```python
from build123d import *
from build123d.topology import SkipClean

# Parameters (mm, degrees)
SKETCH1_R    = 19.05
SKETCH1_R_2  = 12.7
TOP_DEPTH    = 12.7
MIDDLE_START = 6.35
SKETCH4_R    = 28.575
SKETCH4_R_2  = 12.7
MIDDLE_DEPTH = 6.35
BOTTOM_START = 12.7
SKETCH5_R    = 15.875
SKETCH5_R_2  = 12.7
BOTTOM_DEPTH = 12.7


with BuildPart() as part:
    # Sketch1 → Top (new body)
    with BuildSketch(Plane(origin=(0, 0, 0), x_dir=(1, 0, 0), z_dir=(0, 1, 0))):
        with Locations(Location((0, 0, 0), (0, 0, 270))):
            Circle(SKETCH1_R)
        with Locations(Location((0, 0, 0), (0, 0, 270))):
            Circle(SKETCH1_R_2, mode=Mode.SUBTRACT)
    extrude(amount=TOP_DEPTH)

    # Sketch4 → Middle (add)
    with SkipClean():  # the faces are left unmerged after this step: merging them gives an invalid solid
        with BuildSketch(Plane.XZ.offset(MIDDLE_START)):
            with Locations(Location((0, 0, 0), (0, 0, 270))):
                Circle(SKETCH4_R)
            with Locations(Location((0, 0, 0), (0, 0, 270))):
                Circle(SKETCH4_R_2, mode=Mode.SUBTRACT)
        extrude(amount=-MIDDLE_DEPTH)

    # Sketch5 → Bottom (add)
    with SkipClean():  # the faces are left unmerged after this step: merging them gives an invalid solid
        with BuildSketch(Plane.XZ.offset(6.35).offset(BOTTOM_START)):
            with Locations(Location((0, 0, 0), (0, 0, 270))):
                Circle(SKETCH5_R)
            with Locations(Location((0, 0, 0), (0, 0, 270))):
                Circle(SKETCH5_R_2, mode=Mode.SUBTRACT)
        extrude(amount=-BOTTOM_DEPTH)


solid = part.part
```
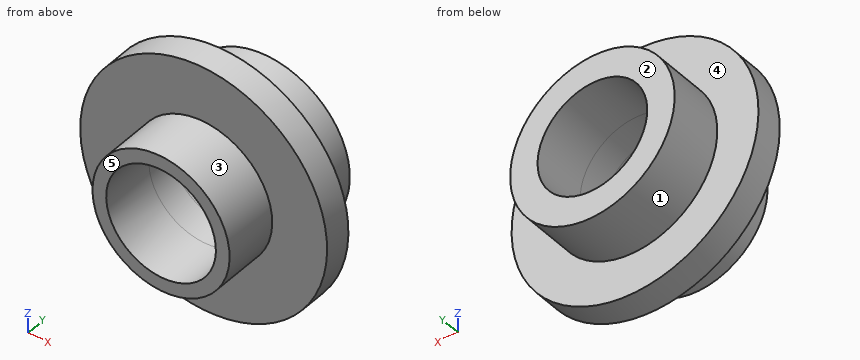
Work out the finished part from the listing and answer in its coordinate system (mm). Face numbers are marked on the shaded views. A direction names the side the tool comes from. Round coordinates to 2 decimals unless told otherwise and drop trailing zeros. Loops run counter-clockwise (first coordinate to the right, second up) from the corner with the lowest first, then second, coordinate; pieces in that order, holes last. Notation, with made-up numbers: M 56.5,60 L 75.5,60 A28 ccw 75.5,94 Z; hole C 67,-28.75 d1. An arc over 180 degrees is marked long. Use CSV: the item, a comma, the result in double quotes.
Q1. Section B-B, the plane z = 0 is taken. Determine the outline of the cut face in (x, y) (3 decimals), then the cut area to 3 significant figures.
Determined:
outline,"M -28.575,-6.35 L -15.875,-6.35 L -15.875,-19.05 L -12.7,-19.05 L -12.7,12.7 L -19.05,12.7 L -19.05,0 L -28.575,0 Z; M 12.7,-19.05 L 15.875,-19.05 L 15.875,-6.35 L 28.575,-6.35 L 28.575,0 L 19.05,0 L 19.05,12.7 L 12.7,12.7 Z"
area,"444 mm2"
Q2. Each of these flat-tipped pins is pushed along its axis until it touches: pin 1 (15 mm diameter, centred on x = 0, z = 0, fed in from -Y); pin 2 (12 mm diameter, centred on x = -12.5, y = -0.5, fed in from -Z); pin 3 (3 mm diameter, centred on y = 6, z = -18.5, fed in from +X); pin 4 (3 mm diameter, centred on x = -5, y = -16, fed in from -Z). Where does it stop, or does it pass through?
Determined:
pin 1,"through"
pin 2,"z = -27.83"
pin 3,"x = 8.6"
pin 4,"z = -15.48"
Q3. Consider L1, parallel to X at y = 8, z = 0; L2, parallel to X at y = -1.25, z = 0 (3 decimals); L3, parallel to Y at x = -7, z = 16.5. Determine where each line is inside the solid, lowest interval first.
Determined:
L1,"-19.05 to -12.7, 12.7 to 19.05"
L2,"-28.575 to -12.7, 12.7 to 28.575"
L3,"-6.35 to 12.7"
Q4. Section A-A, the plane x = 0 is taken. Determine the outline of the cut face in (y, z) (3 decimals), then the cut area to 3 significant figures.
Determined:
outline,"M -19.05,-15.875 L -6.35,-15.875 L -6.35,-28.575 L 0,-28.575 L 0,-19.05 L 12.7,-19.05 L 12.7,-12.7 L -19.05,-12.7 Z; M -19.05,12.7 L 12.7,12.7 L 12.7,19.05 L 0,19.05 L 0,28.575 L -6.35,28.575 L -6.35,15.875 L -19.05,15.875 Z"
area,"444 mm2"
Q5. Section D-D, the plane x = -14 is taken. Determine the outline of the cut face in (y, z), then the cut area to 3 significant figures.
Determined:
outline,"M -19.05,-7.48 L -6.35,-7.48 L -6.35,-24.91 L 0,-24.91 L 0,-12.92 L 12.7,-12.92 L 12.7,12.92 L 0,12.92 L 0,24.91 L -6.35,24.91 L -6.35,7.48 L -19.05,7.48 Z"
area,"835 mm2"
Q6. The mould has two halves that part along Z. Classify the marked faces 1 and 2: pulls with the +Z half, pulls with the -Z half, needs draft (parallel to the pull), parting line crosses it, or undercut.
Determined:
face 1,"parting line crosses it"
face 2,"needs draft"
Q7. A tool of negligible diameter and unlimited length cuts with its end or side. For the marked faces 3, 4 and 5, from which of +Z, -Z, +X, -X, +Y, -Y can it reach the whole face along a straight path? Write none if from no direction.
Determined:
face 3,"-Y"
face 4,"+Y"
face 5,"+Z, -Z, +X, -X, -Y"
Q8. Section C-C, the plane y = -15 is taken. Determine the outline of the cut face in (x, z) (3 decimals).
Determined:
outline,"C 0,0 d31.75; hole C 0,0 d25.4"
